For this review, take the finished solid that the model builds, in its own axes (mm). Face numbers are marked on the shaded views. A direction names the side the tool comes from. Coordinates: 2 decimals unless noted, no trailing zeros. Order: outer loops, then holes, each group sorted by start corner. A loop starts at its lowest first (then second) coordinate and runs counter-clockwise, first axis right, second up.
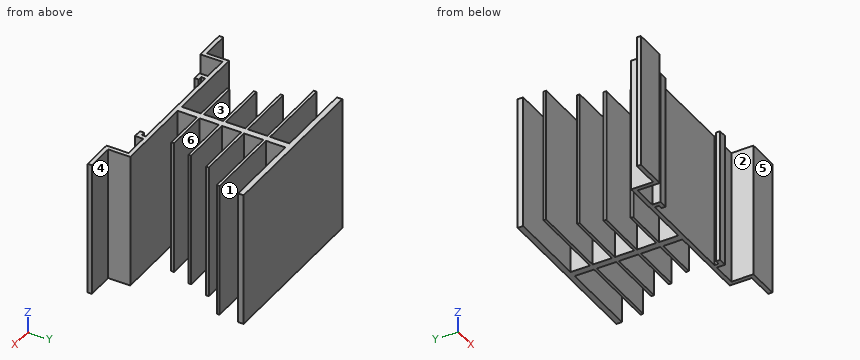
from build123d import *

# Parameters (mm, degrees)
SKETCH1_W           = 60.5
SKETCH1_H           = 42.5
BOSS_EXTRUDE1_DEPTH = 24.5
BOSS_EXTRUDE2_DEPTH = 49
CUT_EXTRUDE1_DEPTH  = 50


with BuildPart() as part:
    # Sketch1 → Boss-Extrude1 (new body, symmetric)
    with BuildSketch(Plane.XY):
        Rectangle(SKETCH1_W, SKETCH1_H)
    extrude(amount=BOSS_EXTRUDE1_DEPTH, both=True)

    # Sketch2 → Boss-Extrude2 (add)
    with BuildSketch(Plane.XY.offset(24.5)):
        Polygon((-30.25, -21.25), (-30.25, -27.75), (-40.25, -27.75), (-40.25, -29.25), (-28.75, -29.25), (-28.75, -21.25), align=None)
        Polygon((-19.75, -21.25), (-19.75, -24.25), (-16.75, -24.25), (-16.75, -22.75), (-18.25, -22.75), (-18.25, -21.25), align=None)
    boss_extrude2 = extrude(amount=-BOSS_EXTRUDE2_DEPTH)

    # Sketch3 → Cut-Extrude1 (cut, through all)
    with BuildSketch(Plane.XY.offset(24.5)):
        Polygon((-30.25, 19.25), (-30.25, -19.75), (-1.25, -19.75), (-1.25, -12.75), (-17, -12.75), (-17, -11.75), (-1.25, -11.75), (-1.25, -4.75), (-20, -4.75), (-20, -3.75), (-1.25, -3.75), (-1.25, 3.25), (-22.75, 3.25), (-22.75, 4.25), (-1.25, 4.25), (-1.25, 11.25), (-29.75, 11.25), (-29.75, 12.25), (-1.25, 12.25), (-1.25, 19.25), align=None)
    cut_extrude1 = extrude(amount=-CUT_EXTRUDE1_DEPTH, mode=Mode.SUBTRACT)

    # Mirror1: Boss-Extrude2, Cut-Extrude1 across plane
    add(boss_extrude2.mirror(Plane(origin=(0, 0, 0), x_dir=(0, 0, 1), z_dir=(1, 0, 0))))
    add(cut_extrude1.mirror(Plane(origin=(0, 0, 0), x_dir=(0, 0, 1), z_dir=(1, 0, 0))), mode=Mode.SUBTRACT)


solid = part.part
1. Take a section at B-B, the plane y = 14. Give the boundary of the cut face in (x, z), plus the area to 4 significant figures.
Answer below:
outline: (-1.25, -24.5) - (1.25, -24.5) - (1.25, 24.5) - (-1.25, 24.5) - close
area: 122.5 mm2
2. Take a section at A-A, the plane x = 5. Give the boundary of the cut face in (y, z).
Answer below:
outline: (-21.25, -24.5) - (-19.75, -24.5) - (-19.75, 24.5) - (-21.25, 24.5) - close; (-12.75, -24.5) - (-11.75, -24.5) - (-11.75, 24.5) - (-12.75, 24.5) - close; (-4.75, -24.5) - (-3.75, -24.5) - (-3.75, 24.5) - (-4.75, 24.5) - close; (3.25, -24.5) - (4.25, -24.5) - (4.25, 24.5) - (3.25, 24.5) - close; (11.25, -24.5) - (12.25, -24.5) - (12.25, 24.5) - (11.25, 24.5) - close; (19.25, -24.5) - (21.25, -24.5) - (21.25, 24.5) - (19.25, 24.5) - close
3. Machinability: for the marked faces 3, 4, 5 and 6, which of the approach directions +Z, -Z, +X, -X, +Y, -Y give a long, thin tool a straight path to every point of the face, cutting with its end or side? Answer none if there is none.
Answer below:
face 3: +Z, -Z, -X
face 4: +Z, -Z, +X, +Y
face 5: +Z, -Z, +X, -X, -Y
face 6: +Z, -Z, +X
4. Clearance check with flat-ended pins moving along their axes: pin 1 Ø0.5 at (y, z) = (3.5, 12) entering from -X; pin 2 Ø1.6 at (y, z) = (20.5, -4) entering from -X; pin 3 Ø8 at (y, z) = (-13, 3) entering from +X. State where each tip first meets the part, or that it passes through.
Answer below:
pin 1: stops at x = -22.75
pin 2: stops at x = -30.25
pin 3: stops at x = 17
5. Take a section at C-C, the plane x = 33. Give the boundary of the cut face in (y, z), plus the area to 3 significant figures.
Answer below:
outline: (-29.25, -24.5) - (-27.75, -24.5) - (-27.75, 24.5) - (-29.25, 24.5) - close
area: 73.5 mm2
6. The part is to be moulded in two halves that separate along X. For the marked faces 1 and 2, say which applies: +X half, -X half, draft (parallel to the pull), parting line (faces both ways), or undercut.
Answer below:
face 1: draft
face 2: undercut
7. To check wall thickness, follow L1, parallel to Y at x = 22, z = -7.5; L2, parallel to Y at x = -3, z = 11; L3, parallel to X at y = -22, z = 15. State the ranges of each line that lie inside material, in increasing order.
Answer below:
L1: y = -21.25 to -19.75, 3.25 to 4.25, 11.25 to 12.25, 19.25 to 21.25
L2: y = -21.25 to -19.75, -12.75 to -11.75, -4.75 to -3.75, 3.25 to 4.25, 11.25 to 12.25, 19.25 to 21.25
L3: x = -30.25 to -28.75, -19.75 to -18.25, 18.25 to 19.75, 28.75 to 30.25
